Geometry: see drawing. Coordinates: mm, zero at the bounding-box minimum. A direction names the side the tool comes from. Coordinates: 2 decimals unless noted, no trailing zeros. Write each loop counter-clockwise with the first axis right and the second up, starting at its lowest first coordinate (ties: lowest second). Pieces come first, ordered by that corner, then holes. Notation, with made-up numbers: (47.25, -37) -> (70.25, -37) arc R24 cw to (70.25, -11) -> close; hole circle Ø5 at (52.25, 19.5). An arc over 180 degrees is marked (long way). Use one line per item in the form item = value. Start each with the question number.
(1) Set-up query: the marked faces 1 and 2. Return all of +Z, -Z, +X, -X, +Y, -Y with unobstructed straight access to the full face (end or side cutting, diameter ignored); none if empty.
(2) First-contact query: pin 1 (0.9 mm diameter, centred on y = 11, z = 17, fed in from -X); pin 2 (1.5 mm diameter, centred on x = 10, y = 6, fed in from +Z); pin 3 (2 mm diameter, centred on x = 17.5, y = 7.5, fed in from +Z) (1 decimal). Flat tips, straight axial feed; report the tip coordinate or a pass-through.
(3) Pull-direction query (Z, two-part tool) for the marked faces 3, 4 and 5; classes: released by +Z, released by -Z, zero draft, split by the parting line, or undercut.
(4) Cut plane A-A on x = 14. Return the cut outline in (y, z).
(5) Cut plane B-B on y = 12.75. Return the cut outline in (x, z) (1 decimal), plus the area to 3 significant figures.
(6) Cut plane C-C on z = 14. Return the cut outline in (x, y), plus the area to 3 significant figures.
(7) Ray query, line 1 along X through (y, z) = (5.25, 14); line 2 along Y through (x, z) = (7, 7.25). Return the intervals inside material, ascending.
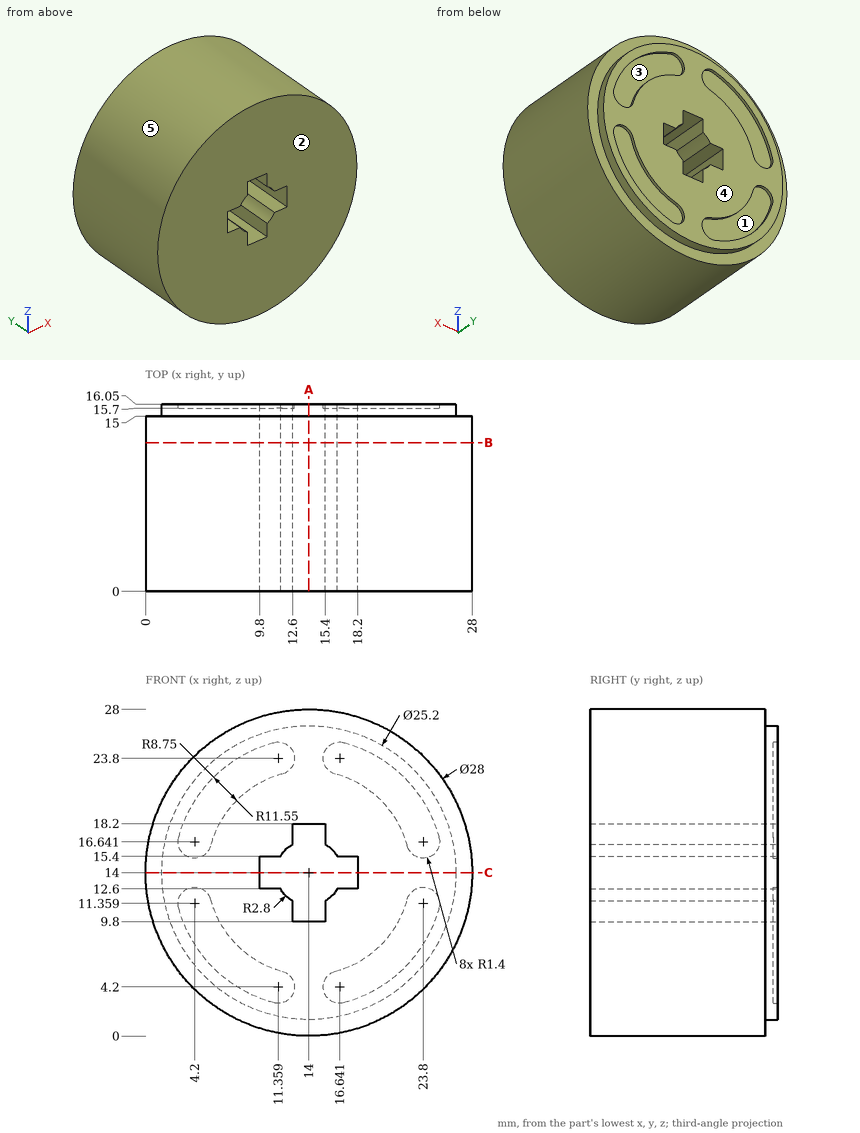
Values:
q1.face_1 = +Y
q1.face_2 = +Z, -Z, +X, -X, -Y
q2.pin_1 = 0.23
q2.pin_2 = 27.62
q2.pin_3 = 27.8
q3.face_3 = undercut
q3.face_4 = zero draft
q3.face_5 = split by the parting line
q4.outline = (0, 0) -> (15, 0) -> (15, 1.4) -> (16.05, 1.4) -> (16.05, 9.8) -> (0, 9.8) -> close; (0, 18.2) -> (16.05, 18.2) -> (16.05, 26.6) -> (15, 26.6) -> (15, 28) -> (0, 28) -> close
q5.outline = circle Ø28 at (14, 14); hole (9.8, 12.6) -> (11.6, 12.6) arc R2.8 ccw to (12.6, 11.6) -> (12.6, 9.8) -> (15.4, 9.8) -> (15.4, 11.6) arc R2.8 ccw to (16.4, 12.6) -> (18.2, 12.6) -> (18.2, 15.4) -> (16.4, 15.4) arc R2.8 ccw to (15.4, 16.4) -> (15.4, 18.2) -> (12.6, 18.2) -> (12.6, 16.4) arc R2.8 ccw to (11.6, 15.4) -> (9.8, 15.4) -> close
q5.area = 574 mm2
q6.outline = (0, 0) -> (9.8, 0) -> (9.8, 16.05) -> (1.4, 16.05) -> (1.4, 15) -> (0, 15) -> close; (18.2, 0) -> (28, 0) -> (28, 15) -> (26.6, 15) -> (26.6, 16.05) -> (18.2, 16.05) -> close
q6.area = 312 mm2
q7.line_1 = 0 to 9.8, 18.2 to 28
q7.line_2 = 0 to 15.7
